For this review, take the finished solid that the model builds, in its own axes (mm). A direction names the side the tool comes from. Coordinates: 2 decimals unless noted, no trailing zeros. Write each loop counter-clockwise with the first axis right and the second up, starting at its lowest first coordinate (ties: lowest second). Pieces come first, ordered by that corner, then holes. Notation, with made-up numbers: M -2,-26 L 26,-26 A24 cw 26,12 Z; hole C 57.5,-36 d2. An arc over 180 degrees is marked long. One line per question, with ' | ' between items.
from build123d import *

# Parameters (mm, degrees)
F0_W     = 25.4
F0_H     = 254
F1_DEPTH = 25.4
F2_T     = -3.175
F4_DEPTH = 3.175


with BuildPart() as f1:
    # F0 (on Top) → F1 (new body)
    with BuildSketch(Plane.XY):
        with Locations((2.03523, 88.852645)):
            Rectangle(F0_W, F0_H)
    extrude(amount=F1_DEPTH)

    # F2
    f2_openings = [f1.faces().sort_by_distance(p)[0] for p in [
        (2.03523, -38.147355, 12.7),
    ]]
    offset(amount=F2_T, openings=f2_openings)

    # F3 (on face) → F4 (join)
    with BuildSketch(Plane(origin=(-10.66477, 0, 0), x_dir=(0, -1, 0), z_dir=(-1, 0, 0))):
        with BuildLine():
            ThreePointArc((-203.152645, 0), (-194.172389, 3.719744), (-190.452645, 12.7))
            ThreePointArc((-190.452645, 12.7), (-194.172389, 21.680256), (-203.152645, 25.4))
            ThreePointArc((-203.152645, 25.4), (-212.132901, 21.680256), (-215.852645, 12.7))
            ThreePointArc((-215.852645, 12.7), (-212.132901, 3.719744), (-203.152645, 0))
        make_face()
    extrude(amount=F4_DEPTH)


solid = f1.part
1. Take a section at D-D on z = 20. State the section outline as (x, y) points.
Computed values:
outline: M -13.84,192.76 L -10.66,192.76 L -10.66,-38.15 L -7.49,-38.15 L -7.49,212.68 L 11.56,212.68 L 11.56,-38.15 L 14.74,-38.15 L 14.74,215.85 L -10.66,215.85 L -10.66,213.54 L -13.84,213.54 Z
2. Draft analysis for pull direction X (two halves, no side actions). For faces 1 (the flat face through (-9, -38.147, 13)), 2 (the flat face through (-7.49, 86, 13)), 3 (the flat face through (-10.665, 213, 3)), 4 (the flat face through (11.56, 86, 13)), state which applies: pulls with the +X half, pulls with the -X half, needs draft (parallel to the pull), parting line crosses it, or undercut.
Computed values:
face 1: needs draft | face 2: undercut | face 3: pulls with the -X half | face 4: undercut
3. Machinability: for faces 5 (the flat face through (-10.665, 213, 23)), 6 (the flat face through (2, 89, 22.225)), 7 (the flat face through (2, 91, 0)), which of the approach directions +Z, -Z, +X, -X, +Y, -Y give a long, thin tool a straight path to every point of the face, cutting with its end or side? Answer none if there is none.
Computed values:
face 5: +Z, -X, +Y | face 6: -Y | face 7: -Z, +X, -X, +Y, -Y
4. For line 1 along Z through (x, y) = (6.5, 198) (3 decimals); line 2 along X through (y, z) = (162.5, 21.25); line 3 along Y through (x, z) = (2, 16.5), list the stretches that pass through material, from the lowest coordinate up.
Computed values:
line 1: z = 0 to 3.175, 22.225 to 25.4 | line 2: x = -10.66 to -7.49, 11.56 to 14.74 | line 3: y = 212.68 to 215.85
5. Take a section at B-B on x = 1.75. State the section outline as (y, z) points (3 decimals), plus the area to 3 significant figures.
Computed values:
outline: M -38.147,0 L 215.853,0 L 215.853,25.4 L -38.147,25.4 L -38.147,22.225 L 212.678,22.225 L 212.678,3.175 L -38.147,3.175 Z | area: 1,670 mm2
6. Clearance check with flat-ended pins moving along their axes: P1, Ø10, axis at y = 128, z = 9.5, coming from the -X side; P2, Ø3, axis at x = 1, z = 17, coming from the -Y side. State where each tip first meets the part, or that it passes through.
Computed values:
P1: stops at x = -10.66 | P2: stops at y = 212.68
7. Take a section at C-C on z = 8. State the section outline as (x, y) points.
Computed values:
outline: M -13.84,191.35 L -10.66,191.35 L -10.66,-38.15 L -7.49,-38.15 L -7.49,212.68 L 11.56,212.68 L 11.56,-38.15 L 14.74,-38.15 L 14.74,215.85 L -10.66,215.85 L -10.66,214.95 L -13.84,214.95 Z
8. Take a section at A-A on y = 98. State the section outline as (x, z) points (3 decimals), plus the area to 3 significant figures.
Computed values:
outline: M -10.665,0 L 14.735,0 L 14.735,25.4 L -10.665,25.4 Z; hole M -7.49,3.175 L 11.56,3.175 L 11.56,22.225 L -7.49,22.225 Z | area: 282 mm2
